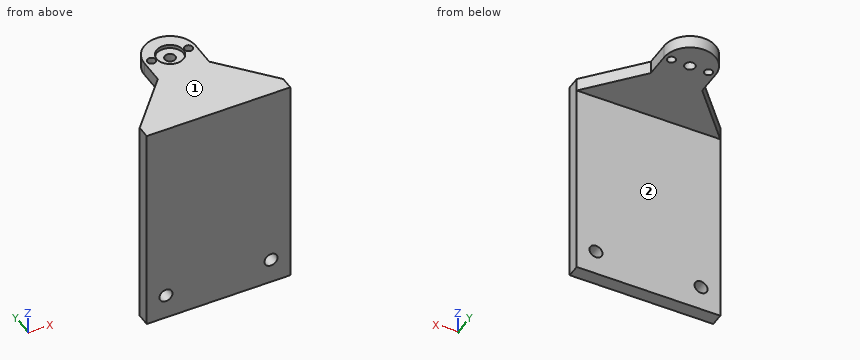
Autodesk Inventor part; units mm, degrees
ref_plane "YZ Plane" through (0, 0, 0) normal (1, 0, 0) x (0, 1, 0)
ref_plane "XZ Plane" through (0, 0, 0) normal (0, 1, 0) x (-1, 0, 0)
ref_plane "XY Plane" through (0, 0, 0) normal (0, 0, 1) x (1, 0, 0)
sketch "Sketch1" plane through (0, 0, 0) normal (0, 0, 1) x (1, 0, 0)
  arc A0 (3.5804, 13.0349) -> (-21.4196, 13.0349) centre (-8.9196, 13.0349) ccw
  line L0 (-21.4196, 13.0349) -> (-21.4196, -24.5571)
  line L1 (-21.4196, -24.5571) -> (3.5804, -24.5571)
  line L2 (3.5804, 13.0349) -> (3.5804, -24.5571)
  circle A1 centre (-8.9196, 13.0349) radius 2.54
  point P0 (0, 0)
  dimension "d10" = 5.08
  dimension "d11" = 12.5
  dimension "d12" = 37.592
extrude "Extrusion1" add sketch "Sketch1" along normal blind 6.35
sketch "Sketch2" plane through (0, 0, 6.35) normal (0, 0, 1) x (1, 0, 0)
  circle A0 centre (-8.9196, 13.0349) radius 2.54
  circle A1 centre (-8.9196, 13.0349) radius 6.5
  point P0 (0, 0)
  dimension "d9" = 13
extrude "Extrusion2" cut sketch "Sketch2" against normal blind 1.778
sketch "Sketch4" plane through (-21.4196, -24.5571, 0) normal (0, -1, 0) x (1, 0, 0)
  line L0 (-22.425, 6.35) -> (47.425, 6.35)
  line L1 (47.425, 6.35) -> (47.425, -97.79)
  line L2 (47.425, -97.79) -> (-22.425, -97.79)
  line L3 (-22.425, -97.79) -> (-22.425, 6.35)
  line L4 (0, 0) -> (0, 6.35)
  line L5 (0, 6.35) -> (0, -15.1092)
  line L6 (12.5, -94.4689) -> (12.5, -35.8122)
  line L7 (0, 6.35) -> (25, 6.35)
  point P0 (21.4196, 0)
  dimension "d15" = 12.5
  dimension "d16" = 69.85
  dimension "d17" = 104.14
extrude "Extrusion5" add sketch "Sketch4" along normal blind 6.35
sketch "Sketch5" plane through (0, 0, 6.35) normal (0, 0, 1) x (1, 0, 0)
  line L0 (-43.8446, -24.5571) -> (-43.8446, -30.9071)
  line L1 (-21.4196, -24.5571) -> (-43.8446, -24.5571)
  line L2 (-43.8446, -24.5571) -> (-21.4196, -24.5571)
  line L3 (-21.4196, -24.5571) -> (-21.4196, 0.8429)
  line L4 (-21.4196, 13.0349) -> (-21.4196, -24.5571)
  line L5 (-43.8446, -24.5571) -> (-21.4196, 0.8429)
  line L6 (26.0054, -24.5571) -> (3.5804, -24.5571)
  line L7 (26.0054, -24.5571) -> (3.5804, 0.8429)
  line L8 (3.5804, 0.8429) -> (3.5804, -24.5571)
  line L9 (3.5804, -24.5571) -> (26.0054, -24.5571)
  point P0 (0, 0)
  dimension "d20" = 25.4
  dimension "d21" = 25.4
extrude "Extrusion6" add sketch "Sketch5" against normal blind 6.35
sketch "Sketch6" plane through (0, 0, 0) normal (0, 0, -1) x (-1, 0, 0)
  circle A0 centre (8.9196, 13.0349) radius 2.54
  line L0 (8.9196, 13.0349) -> (8.9196, 0.8013)
  circle A1 centre (17.9196, 13.0349) radius 2
  circle A2 centre (-0.0804, 13.0349) radius 2
  point P0 (0, 0)
  dimension "d24" = 18
  dimension "d25" = 4
extrude "Extrusion7" cut sketch "Sketch6" against normal through all contours A1 | A2
sketch "Sketch7" plane through (-21.4196, -30.9071, 0) normal (0, -1, 0) x (1, 0, 0)
  circle A0 centre (-13.0588, -85.598) radius 3.175
  line L0 (12.5, -78.7871) -> (12.5, -99.3381)
  circle A1 centre (38.0588, -85.598) radius 3.175
  line L1 (47.425, 6.35) -> (-22.425, 6.35)
  point P0 (21.4196, 0)
  dimension "d28" = 6.35
  dimension "d29" = 51.1175
  dimension "d30" = 91.948
extrude "Extrusion8" cut sketch "Sketch7" against normal through all
properties part number "encoder_mount"
Source: CAD feature listing. Evaluate the final solid. Frame: model axes, mm. Face numbers are marked on the shaded views. A direction names the side the tool comes from. Coordinates: 2 decimals unless noted, no trailing zeros. Loops run counter-clockwise (first coordinate to the right, second up) from the corner with the lowest first, then second, coordinate; pieces in that order, holes last. Notation, with made-up numbers: (-34, 18.5) -> (-14, 18.5) arc R19 ccw to (-14, 41.5) -> close; hole circle Ø8 at (-22.75, 46). An arc over 180 degrees is marked (long way). Answer in a Markdown table with one row per item. Add a question column.
Q1. Contact query for flat-ended pins moving along their axis: pin 1 Ø2 at (x, y) = (-20, -1.5) entering from -Z; pin 2 Ø3 at (y, z) = (10, 3.5) entering from +X; pin 3 Ø5 at (y, z) = (6.5, 4.5) entering from -X; pin 4 Ø4.5 at (x, y) = (-8.92, 13.03) entering from +Z. Output: stop coordinate, or through.
Q2. Section A-A on x = -35.5. Return the cut outline in (y, z), and give its area (3 significant figures).
Q3. Reachability of the marked faces 1 and 2 from +Z, -Z, +X, -X, +Y, -Y: full face, straight path, thin tool, end or side. Return the list, or none.
Q4. Section D-D on y = 21.5. Return the cut outline in (x, z), and give its area (3 significant figures).
Q5. Section C-C on z = -59. Return the cut outline in (x, y).
Q6. Ray query, line 1 along Z through (x, y) = (-18, 21); line 2 along Y through (x, z) = (-6, -47.5); line 3 along Z through (x, y) = (-12.5, 12). Return the intervals inside material, ascending.
Q7. Section B-B on x = -13. Return the cut outline in (y, z).
Computed values:
| question | item | result |
|---|---|---|
| 1 | pin 1 | stops at z = 0 |
| 1 | pin 2 | stops at x = 3.58 |
| 1 | pin 3 | stops at x = -21.42 |
| 1 | pin 4 | passes through |
| 2 | outline | (-30.91, -97.79) -> (-24.56, -97.79) -> (-24.56, -88.6) -> (-30.91, -88.6) -> close; (-30.91, -82.59) -> (-24.56, -82.59) -> (-24.56, 0) -> (-15.11, 0) -> (-15.11, 6.35) -> (-30.91, 6.35) -> close |
| 2 | area | 683 mm^2 |
| 3 | face 1 | +Z, +X, -X, +Y, -Y |
| 3 | face 2 | -Z, +X, -X, +Y |
| 4 | outline | (-18.12, 0) -> (0.28, 0) -> (0.28, 6.35) -> (-18.12, 6.35) -> close |
| 4 | area | 117 mm^2 |
| 5 | outline | (-43.84, -30.91) -> (26.01, -30.91) -> (26.01, -24.56) -> (-43.84, -24.56) -> close |
| 6 | line 1 | z = 0 to 6.35 |
| 6 | line 2 | y = -30.91 to -24.56 |
| 6 | line 3 | z = 0 to 4.57 |
| 7 | outline | (-30.91, -97.79) -> (-24.56, -97.79) -> (-24.56, 0) -> (24.85, 0) -> (24.85, 6.35) -> (18.09, 6.35) -> (18.09, 4.57) -> (7.98, 4.57) -> (7.98, 6.35) -> (-30.91, 6.35) -> close |
